The figure shows three views and two pictorial views of one solid part (mm, origin at its lowest corner). Answer the questions. A direction names the side the tool comes from. Give positions to 0.01 mm unless a question says otherwise; leave off trailing zeros. Order: outer loops, then holes, each group sorted by start corner. A loop starts at its lowest first (then second) coordinate and runs counter-clockwise, first axis right, second up. Notation, with made-up numbers: M 16.25,44.5 L 68.25,44.5 A19 cw 68.25,63.5 Z; hole C 42,-14.5 d8. An arc over 180 degrees is marked long. One line per item, written item: value. Start each with the question number.
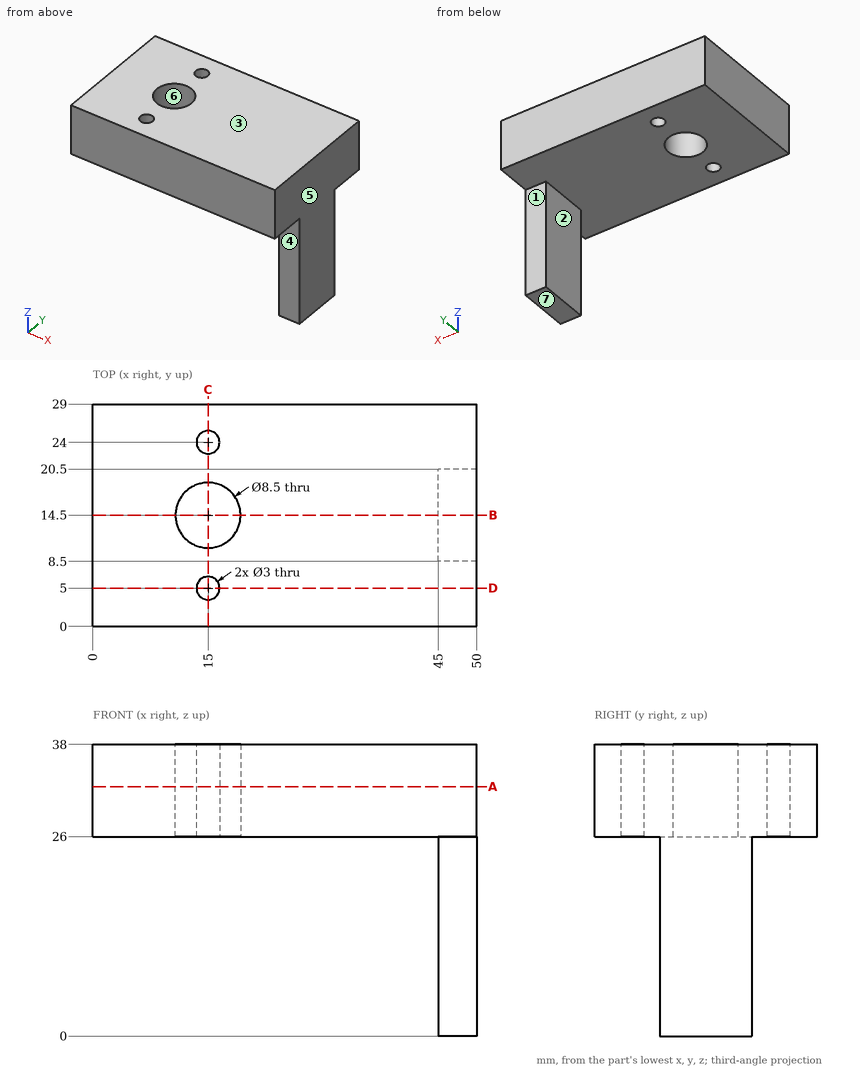
Q1. Find section D-D, the plane y = 5. Give the vertices of the cut face in (x, z), then the cut area to 3 significant figures.
Q2. A tool of negligible diameter and unlimited length cuts with its end or side. For the marked faces 1, 2, 3 and 4, from which of +Z, -Z, +X, -X, +Y, -Y can it reach the whole face along a straight path? Write none if from no direction.
Q3. Find section C-C, the plane x = 15. Give the vertices of the cut face in (y, z), then the cut area to 3 significant figures.
Q4. Determine the mould class of the marked faces 5, 6 and 7 for opening direction X: released by +X, released by -X, zero draft, split by the parting line, or undercut.
Q5. Consider probe 1 along Y at (x, z) = (15, 32.25); probe 2 along Z at (x, y) = (43.5, 23.75); probe 3 along X at (y, z) = (17.5, 30). Determine where each line is inside the solid, lowest interval first.
Q6. Each of these flat-tipped pins is pushed along its axis until it touches: pin 1 (1.5 mm diameter, centred on x = 48, z = 13, fed in from -Y); pin 2 (10 mm diameter, centred on x = 39.5, z = 17, fed in from +Y); pin 3 (11 mm diameter, centred on x = 15, y = 14.5, fed in from -Z); pin 4 (3.5 mm diameter, centred on y = 15.5, z = 13.5, fed in from -X). Where does it stop, or does it pass through?
Q7. Find section B-B, the plane y = 14.5. Give the vertices of the cut face in (x, z), then the cut area to 3 significant figures.
Q8. Find section A-A, the plane z = 32.5. Give the vertices of the cut face in (x, y).
Evaluation:
1. outline: M 0,26 L 13.5,26 L 13.5,38 L 0,38 Z; M 16.5,26 L 50,26 L 50,38 L 16.5,38 Z
1. area: 564 mm2
2. face 1: -Z, +X, -X, +Y
2. face 2: -Z, -X, +Y, -Y
2. face 3: +Z, +X, -X, +Y, -Y
2. face 4: -Z, +X, -X, -Y
3. outline: M 0,26 L 3.5,26 L 3.5,38 L 0,38 Z; M 6.5,26 L 10.25,26 L 10.25,38 L 6.5,38 Z; M 18.75,26 L 22.5,26 L 22.5,38 L 18.75,38 Z; M 25.5,26 L 29,26 L 29,38 L 25.5,38 Z
3. area: 174 mm2
4. face 5: released by +X
4. face 6: undercut
4. face 7: zero draft
5. probe 1: 0 to 3.5, 6.5 to 10.25, 18.75 to 22.5, 25.5 to 29
5. probe 2: 26 to 38
5. probe 3: 0 to 11.99, 18.01 to 50
6. pin 1: y = 8.5
6. pin 2: through
6. pin 3: z = 26
6. pin 4: x = 45
7. outline: M 0,26 L 10.75,26 L 10.75,38 L 0,38 Z; M 19.25,26 L 45,26 L 45,0 L 50,0 L 50,38 L 19.25,38 Z
7. area: 628 mm2
8. outline: M 0,0 L 50,0 L 50,29 L 0,29 Z; hole C 15,14.5 d8.5; hole C 15,5 d3; hole C 15,24 d3
